Source: CAD feature listing. Evaluate the final solid. Frame: model axes, mm. Give positions to 0.01 mm unless a question says otherwise; leave off trailing zeros. Order: outer loops, then holes, each group sorted by start corner. A loop starts at its lowest first (then second) coordinate and runs counter-clockwise, first axis right, second up. Notation, with made-up numbers: M 87,80.5 L 103,80.5 A23 cw 103,102.5 Z; hole C 44.5,-22 d5. An arc over 180 degrees is marked long. Use CSV: the item, a comma, the result in double quotes. Start each with the question number.
Item 1: Section query A-A on x = -87.05. Return loops of the section in (y, z).
Item 2: Ray query, probe 1 along Y at (x, z) = (-120, 0.8); probe 2 along X at (y, z) = (22, 0.35); probe 3 along X at (y, z) = (-28, 1.6). Return the intervals inside material, ascending. Write a range as from..to.
Item 3: Section query B-B on z = 3.4. Return loops of the section in (x, y).
Item 4: First-contact query: pin 1 (8 mm diameter, centred on x = -110, y = 22.5, fed in from +Z); pin 2 (2 mm diameter, centred on x = -104, z = 2.5, fed in from -Y); pin 3 (2 mm diameter, centred on y = -27, z = 1.5, fed in from +X); pin 4 (1.2 mm diameter, centred on y = -25, z = 2.5, fed in from +X). Flat tips, straight axial feed; report the tip coordinate or a pass-through.
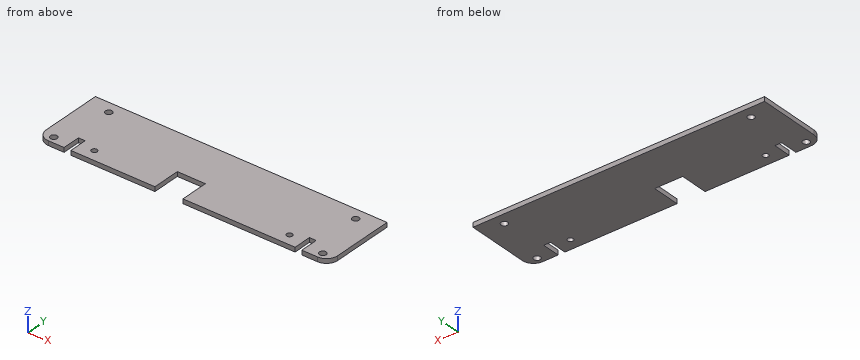
from build123d import *

# Parameters (mm, degrees)
SKETCH1_W           = 260
SKETCH1_H           = 65
BOSS_EXTRUDE2_DEPTH = 4
SKETCH3_R           = 3
CUT_EXTRUDE2_DEPTH  = 135.060620616
FILLET1_R           = 10
SKETCH4_W           = 25
SKETCH4_H           = 25
CUT_EXTRUDE3_DEPTH  = 10
SKETCH5_W           = 6
SKETCH5_H           = 16
CUT_EXTRUDE4_DEPTH  = 135.060620616
SKETCH6_R           = 2.5
CUT_EXTRUDE5_DEPTH  = 135.060620616


with BuildPart() as part:
    # Sketch1 → Boss-Extrude2 (new body)
    with BuildSketch(Plane.XY):
        Rectangle(SKETCH1_W, SKETCH1_H)
    extrude(amount=BOSS_EXTRUDE2_DEPTH)

    # Sketch3 → Cut-Extrude2 (cut, through all)
    with BuildSketch(Plane(origin=(0, 0, 0), x_dir=(-1, 0, 0), z_dir=(0, 0, -1))):
        with Locations((120, -26.5)):
            Circle(SKETCH3_R)
        with Locations((-120, -26.5)):
            Circle(SKETCH3_R)
        with Locations((-110, 22.5)):
            Circle(SKETCH3_R)
        with Locations((110, 22.5)):
            Circle(SKETCH3_R)
    extrude(amount=-CUT_EXTRUDE2_DEPTH, mode=Mode.SUBTRACT)

    # Fillet1
    fillet1_edges = [part.edges().sort_by_distance(p)[0] for p in [
        (130, -32.5, 2),
        (-130, -32.5, 2),
    ]]
    fillet(fillet1_edges, radius=FILLET1_R)

    # Sketch4 → Cut-Extrude3 (cut)
    with BuildSketch(Plane(origin=(0, 0, 0), x_dir=(-1, 0, 0), z_dir=(0, 0, -1))):
        with Locations((12.5, -20)):
            Rectangle(SKETCH4_W, SKETCH4_H)
    extrude(amount=-CUT_EXTRUDE3_DEPTH, mode=Mode.SUBTRACT)

    # Sketch5 → Cut-Extrude4 (cut, through all)
    with BuildSketch(Plane(origin=(0, 0, 0), x_dir=(-1, 0, 0), z_dir=(0, 0, -1))):
        with Locations((-103, -24.5)):
            Rectangle(SKETCH5_W, SKETCH5_H)
        with Locations((103, -24.5)):
            Rectangle(SKETCH5_W, SKETCH5_H)
    extrude(amount=-CUT_EXTRUDE4_DEPTH, mode=Mode.SUBTRACT)

    # Sketch6 → Cut-Extrude5 (cut, through all)
    with BuildSketch(Plane(origin=(0, 0, 0), x_dir=(-1, 0, 0), z_dir=(0, 0, -1))):
        with Locations((87.05, -22.5)):
            Circle(SKETCH6_R)
        with Locations((-87.05, -22.5)):
            Circle(SKETCH6_R)
    extrude(amount=-CUT_EXTRUDE5_DEPTH, mode=Mode.SUBTRACT)


solid = part.part
Verdict:
1,outline,"M -32.5,0 L -25,0 L -25,4 L -32.5,4 Z; M -20,0 L 32.5,0 L 32.5,4 L -20,4 Z"
2,probe 1,"-32.5..-29.5, -23.5..32.5"
2,probe 2,"-130..-112.96, -107.04..107.04, 112.96..130"
2,probe 3,"-128.35..-122.6, -117.4..-106, -100..-25, 0..100, 106..117.4, 122.6..128.35"
3,outline,"M -130,-22.5 A10 ccw -120,-32.5 L -106,-32.5 L -106,-16.5 L -100,-16.5 L -100,-32.5 L -25,-32.5 L -25,-7.5 L 0,-7.5 L 0,-32.5 L 100,-32.5 L 100,-16.5 L 106,-16.5 L 106,-32.5 L 120,-32.5 A10 ccw 130,-22.5 L 130,32.5 L -130,32.5 Z; hole C -120,-26.5 d6; hole C -110,22.5 d6; hole C -87.05,-22.5 d5; hole C 87.05,-22.5 d5; hole C 110,22.5 d6; hole C 120,-26.5 d6"
4,pin 1,"z = 4"
4,pin 2,"y = -16.5"
4,pin 3,"x = 129.37"
4,pin 4,"x = 129.82"
